Geometry: final body of the model. Coordinates: model frame, mm. Coordinates: 2 decimals unless noted, no trailing zeros. Order: outer loops, then holes, each group sorted by start corner. A loop starts at its lowest first (then second) coordinate and runs counter-clockwise, first axis right, second up. Notation, with made-up numbers: (1, 82.25) -> (55, 82.25) arc R5 ccw to (55, 90.25) -> close; hole circle Ø8 at (-6, -38). An arc over 180 degrees is marked (long way). Answer in a Markdown table with one row per item. Add a question column.
1) Pull-direction query (X, two-part tool) for faces 1 (the face through (150, 0, 6)), 2 (the face through (285.97, 13.85, 6.08)), 3 (the face through (301.7, 1.43, 6.08)); classes: +X half, -X half, draft (parallel to the pull), parting line (faces both ways), or undercut.
2) Section query B-B on x = 283.2. Return the cut outline in (y, z).
3) Section query A-A on y = 15. Return the cut outline in (x, z), then the cut area to 3 significant figures.
4) Contact query for a flat-ended pin moving along its axis: P1, Ø3.5, axis at x = 283.2, y = 15, coming from the -Z side. Output: stop coordinate, or through.
5) Ray query, line 1 (X direction, y = 15.5, z = 2.75); line 2 (Y direction, x = 283.2, z = 8.75); line 3 (X direction, y = 1.25, z = 9.5). Return the intervals inside material, ascending. Write a range as from..to.
Autodesk Inventor part; units mm, degrees
ref_plane "YZ Plane" through (0, 0, 0) normal (1, 0, 0) x (0, 1, 0)
ref_plane "XZ Plane" through (0, 0, 0) normal (0, 1, 0) x (-1, 0, 0)
ref_plane "XY Plane" through (0, 0, 0) normal (0, 0, 1) x (1, 0, 0)
sketch "Sketch1" plane through (0, 0, 0) normal (0, 0, 1) x (1, 0, 0)
  line L0 (0, 0) -> (303.2, 0)
  line L1 (303.2, 0) -> (303.2, 30)
  line L2 (303.2, 30) -> (0, 30)
  line L3 (0, 30) -> (0, 0)
  dimension "d0" = 303.2
  dimension "d1" = 30
extrude "Extrusion1" add sketch "Sketch1" along normal blind 12
fillet "Fillet1" radius 5 1 edges at (0, 30, 6)
fillet "Fillet2" radius 5 3 edges at (303.2, 30, 6) (303.2, 0, 6) (0, 0, 6)
sketch "Sketch2" plane through (0, 0, 12) normal (0, 0, 1) x (1, 0, 0)
  line L0 (0, 25) -> (0, 5)
  line L1 (0, 15) -> (20, 15)
  circle A0 centre (20, 15) radius 3
  line L2 (5, 0) -> (298.2, 0)
  line L3 (151.6, 0) -> (151.6, 30)
  line L4 (298.2, 30) -> (5, 30)
  circle A1 centre (283.2, 15) radius 3
  point P0 (0, 0)
  dimension "d6" = 20
  dimension "d7" = 6
extrude "Extrusion2" cut sketch "Sketch2" against normal through all
properties part number "Fourbar-Coupler"
Result:
| question | item | result |
|---|---|---|
| 1 | face 1 | draft |
| 1 | face 2 | undercut |
| 1 | face 3 | +X half |
| 2 | outline | (0, 0) -> (12, 0) -> (12, 12) -> (0, 12) -> close; (18, 0) -> (30, 0) -> (30, 12) -> (18, 12) -> close |
| 3 | outline | (0, 0) -> (17, 0) -> (17, 12) -> (0, 12) -> close; (23, 0) -> (280.2, 0) -> (280.2, 12) -> (23, 12) -> close; (286.2, 0) -> (303.2, 0) -> (303.2, 12) -> (286.2, 12) -> close |
| 3 | area | 3,490 mm2 |
| 4 | P1 | through |
| 5 | line 1 | 0..17.04, 22.96..280.24, 286.16..303.2 |
| 5 | line 2 | 0..12, 18..30 |
| 5 | line 3 | 1.69..301.51 |
